The model under review builds one solid part; all positions refer to its coordinate system, in mm. Give positions to 0.01 mm unless a question says otherwise; leave off trailing zeros. Write each loop counter-clockwise with the first axis right and the second up, starting at its lowest first coordinate (ties: lowest second). Pieces come first, ordered by that corner, then holes. Notation, with made-up numbers: (-2.5, 65.5) - (15.5, 65.5) arc R19 ccw to (15.5, 88.5) - close; hole circle Ø2 at (16.25, 57). An arc over 180 degrees is marked (long way). One line per question, with ' | ' between items. Start each with the question number.
```python
from build123d import *

# Parameters (mm, degrees)
F0_R     = 26.416
F1_DEPTH = 3.175


with BuildPart() as f1:
    # F0 (on Top) → F1 (new body)
    with BuildSketch(Plane.XY):
        Circle(F0_R)
        with BuildLine():
            ThreePointArc((-11.980964, -8.7503), (-18.222779, -9.57205), (-12.406334, -7.1628))
            ThreePointArc((-12.406334, -7.1628), (-12.08915, -7.92855), (-11.980964, -8.7503))
        make_face(mode=Mode.SUBTRACT)
        with BuildLine():
            ThreePointArc((3.175, -17.5006), (-2.245064, -19.745664), (0, -14.3256))
            ThreePointArc((0, -14.3256), (2.245064, -15.255536), (3.175, -17.5006))
        make_face(mode=Mode.SUBTRACT)
        with BuildLine():
            ThreePointArc((18.330964, -8.7503), (14.334214, -11.817114), (12.406334, -7.1628))
            ThreePointArc((12.406334, -7.1628), (15.977715, -5.683486), (18.330964, -8.7503))
        make_face(mode=Mode.SUBTRACT)
        with BuildLine():
            ThreePointArc((-11.980964, 8.7503), (-12.08915, 7.92855), (-12.406334, 7.1628))
            ThreePointArc((-12.406334, 7.1628), (-18.222779, 9.57205), (-11.980964, 8.7503))
        make_face(mode=Mode.SUBTRACT)
        with BuildLine():
            ThreePointArc((10.822546, 6.2484), (12.070982, 3.23441), (12.4968, 0))
            ThreePointArc((12.4968, 0), (12.070982, -3.23441), (10.822546, -6.2484))
            ThreePointArc((10.822546, -6.2484), (6.2484, -10.822546), (0, -12.4968))
            ThreePointArc((0, -12.4968), (-6.2484, -10.822546), (-10.822546, -6.2484))
            ThreePointArc((-10.822546, -6.2484), (-12.4968, 0), (-10.822546, 6.2484))
            ThreePointArc((-10.822546, 6.2484), (-6.2484, 10.822546), (0, 12.4968))
            ThreePointArc((0, 12.4968), (6.2484, 10.822546), (10.822546, 6.2484))
        make_face(mode=Mode.SUBTRACT)
        with BuildLine():
            ThreePointArc((18.330964, 8.7503), (15.977715, 5.683486), (12.406334, 7.1628))
            ThreePointArc((12.406334, 7.1628), (14.334214, 11.817114), (18.330964, 8.7503))
        make_face(mode=Mode.SUBTRACT)
        with BuildLine():
            ThreePointArc((3.175, 17.5006), (2.245064, 15.255536), (0, 14.3256))
            ThreePointArc((0, 14.3256), (-2.245064, 19.745664), (3.175, 17.5006))
        make_face(mode=Mode.SUBTRACT)
    extrude(amount=F1_DEPTH)


solid = f1.part
```
Item 1: Take a section at C-C (y = 10). Give the boundary of the cut face in (x, z) (3 decimals), plus the area to 3 significant figures.
Item 2: Clearance check with a flat-ended pin moving along its axis: P1, Ø5, axis at x = 15.16, y = -8.75, coming from the +Z side. State where the tip first meets the part, or that it passes through.
Item 3: For probe 1 along Y at (x, z) = (17.5, 1.5); probe 2 along X at (y, z) = (6, 1.65); probe 3 along X at (y, z) = (7, 0.4), list the stretches that pass through material, from the lowest coordinate up.
Item 4: The part is to be moulded in two halves that separate along Z. For faces 1 (the flat face through (5.5, -11.4, 0)), 2 (the cylindrical face through (24.4, -10.12, 1.57)), 3 (the flat face through (5.5, -11.4, 3.175)), say which applies: +Z half, -Z half, draft (parallel to the pull), parting line (faces both ways), or undercut.
Item 5: Take a section at D-D (x = -7.5). Give the boundary of the cut face in (y, z) (3 decimals).
Item 6: Take a section at A-A (z = 1.25). Give the boundary of the cut face in (x, y) (3 decimals).
Item 7: Take a section at B-B (x = 10). Give the boundary of the cut face in (y, z) (3 decimals).
Check sheet entries:
1) outline: (-24.45, 0) - (-18.075, 0) - (-18.075, 3.175) - (-24.45, 3.175) - close; (-12.237, 0) - (-7.495, 0) - (-7.495, 3.175) - (-12.237, 3.175) - close; (7.495, 0) - (12.237, 0) - (12.237, 3.175) - (7.495, 3.175) - close; (18.075, 0) - (24.45, 0) - (24.45, 3.175) - (18.075, 3.175) - close | area: 70.6 mm^2
2) P1: passes through
3) probe 1: y = -19.79 to -10.89, -6.61 to 6.61, 10.89 to 19.79 | probe 2: x = -25.73 to -16.74, -13.57 to -10.96, 10.96 to 13.57, 16.74 to 25.73 | probe 3: x = -25.47 to -17.8, -12.51 to -10.35, 10.35 to 12.51, 17.8 to 25.47
4) face 1: -Z half | face 2: draft | face 3: +Z half
5) outline: (-25.329, 0) - (-9.996, 0) - (-9.996, 3.175) - (-25.329, 3.175) - close; (9.996, 0) - (25.329, 0) - (25.329, 3.175) - (9.996, 3.175) - close
6) outline: circle Ø52.832 at (0, 0); hole (-12.406, -7.163) arc R3.175 ccw (long way) to (-11.981, -8.75) arc R3.175 ccw to start; hole (-12.406, 7.163) arc R3.175 ccw to (-11.981, 8.75) arc R3.175 ccw (long way) to start; hole (-10.823, -6.248) arc R12.497 ccw to (0, -12.497) arc R12.497 ccw to (10.823, -6.248) arc R12.497 ccw to (12.497, 0) arc R12.497 ccw to (10.823, 6.248) arc R12.497 ccw to (0, 12.497) arc R12.497 ccw to (-10.823, 6.248) arc R12.497 ccw to start; hole circle Ø6.35 at (0, -17.501); hole circle Ø6.35 at (0, 17.501); hole circle Ø6.35 at (15.156, -8.75); hole circle Ø6.35 at (15.156, 8.75)
7) outline: (-24.45, 0) - (-7.495, 0) - (-7.495, 3.175) - (-24.45, 3.175) - close; (7.495, 0) - (24.45, 0) - (24.45, 3.175) - (7.495, 3.175) - close
